Input: part model. Units: mm. Frame: model coordinates. A direction names the side the tool comes from. Coordinates: 2 decimals unless noted, no trailing zeros. Order: outer loops, then holes, each group sorted by start corner. A loop starts at its lowest first (then second) coordinate and runs counter-clockwise, first axis right, second up. Notation, with made-up numbers: (72.5, 89.25) - (94.5, 89.25) arc R3 ccw to (94.5, 93.25) - close; hole circle Ø5 at (-4.5, -12.5). An arc over 180 degrees is marked (long way). Answer as CSV lines item,"result". Start each with the question number.
Item 1: Section C-C (x = 12.25). Output: boundary loops of the cut face in (y, z), and give its area (3 significant figures).
Item 2: Access query for faces 1 (the flat face through (0, 0, -2.6)), 2 (the flat face through (0, 0, 54.2)), 3 (the cylindrical face through (-5, 0, -1)), 4 (the flat face through (6, 0, 37.8)). Directions: +Z, -Z, +X, -X, +Y, -Y. A direction counts if a zero-diameter tool reaches every point of the face in a straight line with its end or side. Return the directions, or none.
Item 3: Section A-A (y = 0). Output: boundary loops of the cut face in (x, z).
Item 4: Material intervals for line 1 along X through (y, z) = (9.25, 27); line 2 along Z through (x, y) = (-0.25, -7.25); line 3 along Z through (x, y) = (-5.5, -1.5), sorted ascending.
Item 5: Section B-B (z = 15). Output: boundary loops of the cut face in (x, y), and give its area (3 significant figures).
Item 6: First-contact query: pin 1 (3 mm diameter, centred on x = 0, z = -5, fed in from -Y); pin 2 (2 mm diameter, centred on x = 0.42, y = -7.99, fed in from +Z); pin 3 (2 mm diameter, centred on x = 8, z = 2, fed in from -Y). Flat tips, straight axial feed; report the tip coordinate or a pass-through.
Item 7: Draft query along Y for faces 5 (the cylindrical face through (-13.926, 4.385, 23.04)), 6 (the flat face through (0, -11.3, -3)), 7 (the flat face through (0, -11.7, -3)). Return one class per face: +Y half, -Y half, draft (parallel to the pull), parting line (faces both ways), or undercut.
Item 8: Section D-D (z = 46). Output: boundary loops of the cut face in (x, y), and give its area (3 significant figures).
from build123d import *

# Parameters (mm, degrees)
SKETCH_1_R          = 13.85
EXTRUDE_1_DEPTH     = 37.8
SKETCH_2_R          = 5
EXTRUDE_2_DEPTH     = 2.6
EXTRUDE_START       = -2.6
SKETCH_3_R          = 1.15
EXTRUDE_3_DEPTH     = 16.4
EXTRUDE_START_2     = -32.9
SKETCH_4_R          = 14.6
EXTRUDE_4_DEPTH     = 20
EXTRUDE_START_3     = 2.6
SKETCH_5_R          = 5
EXTRUDE_5_DEPTH     = 2.6
SKETCH_6_W          = 2.8
SKETCH_6_H          = 0.4
EXTRUDE_6_DEPTH     = 6.9
SKETCH_7_R          = 1.3
CUT_EXTRUDE_1_DEPTH = 0.45


with BuildPart() as part:
    # ｽｹｯﾁ1 → ﾎﾞｽ - 押し出し1 (new body)
    with BuildSketch(Plane.XY):
        Circle(SKETCH_1_R)
    extrude(amount=EXTRUDE_1_DEPTH)

    # ｽｹｯﾁ2 → ﾎﾞｽ - 押し出し2 (add)
    with BuildSketch(Plane.XY.offset(37.8)):
        Circle(SKETCH_2_R)
    extrude(amount=EXTRUDE_2_DEPTH)

    # ｽｹｯﾁ3 → ﾎﾞｽ - 押し出し3 (add)
    with BuildSketch(Plane.XY.offset(40.4).offset(EXTRUDE_START)):
        Circle(SKETCH_3_R)
    extrude(amount=EXTRUDE_3_DEPTH)

    # ｽｹｯﾁ4 → ﾎﾞｽ - 押し出し4 (add)
    with BuildSketch(Plane(origin=(0, 0, 0), x_dir=(-1, 0, 0), z_dir=(0, 0, -1)).offset(EXTRUDE_START_2)):
        Circle(SKETCH_4_R)
    extrude(amount=EXTRUDE_4_DEPTH)

    # ｽｹｯﾁ5 → ﾎﾞｽ - 押し出し5 (add)
    with BuildSketch(Plane(origin=(0, 0, 0), x_dir=(-1, 0, 0), z_dir=(0, 0, -1)).offset(EXTRUDE_START_3)):
        with Locations(Location((0, 0, 0), (0, 0, 180))):
            Circle(SKETCH_5_R)
    extrude(amount=-EXTRUDE_5_DEPTH)

    # ｽｹｯﾁ6 → ﾎﾞｽ - 押し出し6 (add)
    with BuildSketch(Plane(origin=(0, 0, 0), x_dir=(-1, 0, 0), z_dir=(0, 0, -1))):
        with Locations((0, 11.5)):
            Rectangle(SKETCH_6_W, SKETCH_6_H)
        with Locations((0, -11.5)):
            Rectangle(SKETCH_6_W, SKETCH_6_H)
    extrude(amount=EXTRUDE_6_DEPTH)

    # ｽｹｯﾁ7 → ｶｯﾄ - 押し出し1 (cut)
    with BuildSketch(Plane.XY.offset(37.8)):
        with Locations((-0.41868765, 7.989036278)):
            Circle(SKETCH_7_R)
        with Locations(Location((0.41868765, -7.989036278, 0), (0, 0, 180))):
            Circle(SKETCH_7_R)
    extrude(amount=-CUT_EXTRUDE_1_DEPTH, mode=Mode.SUBTRACT)


solid = part.part
Determined:
1,outline,"(-7.94, 12.9) - (-6.46, 12.9) - (-6.46, 0) - (6.46, 0) - (6.46, 12.9) - (7.94, 12.9) - (7.94, 32.9) - (6.46, 32.9) - (6.46, 37.8) - (-6.46, 37.8) - (-6.46, 32.9) - (-7.94, 32.9) - close"
1,area,"548 mm^2"
2,face 1,"-Z, +X, -X"
2,face 2,"+Z, +X, -X, +Y, -Y"
2,face 3,"-Z"
2,face 4,"+Z"
3,outline,"(-14.6, 12.9) - (-13.85, 12.9) - (-13.85, 0) - (-5, 0) - (-5, -2.6) - (5, -2.6) - (5, 0) - (13.85, 0) - (13.85, 12.9) - (14.6, 12.9) - (14.6, 32.9) - (13.85, 32.9) - (13.85, 37.8) - (5, 37.8) - (5, 40.4) - (1.15, 40.4) - (1.15, 54.2) - (-1.15, 54.2) - (-1.15, 40.4) - (-5, 40.4) - (-5, 37.8) - (-13.85, 37.8) - (-13.85, 32.9) - (-14.6, 32.9) - close"
4,line 1,"x = -11.3 to 11.3"
4,line 2,"z = 0 to 37.35"
4,line 3,"z = 0 to 37.8"
5,outline,"circle Ø29.2 at (0, 0)"
5,area,"670 mm^2"
6,pin 1,"stops at y = -11.7"
6,pin 2,"stops at z = 37.35"
6,pin 3,"stops at y = -11.95"
7,face 5,"parting line"
7,face 6,"undercut"
7,face 7,"-Y half"
8,outline,"circle Ø2.3 at (0, 0)"
8,area,"4.15 mm^2"
